from build123d import *

# Parameters (mm, degrees)
F8_DEPTH  = 16.5
F2_W      = 43
F2_H      = 66
F9_DEPTH  = 15
F4_W      = 6
F4_H      = 6
F4_H_2    = 5
F10_DEPTH = 16.5
F5_W      = 8
F5_H      = 6
F5_W_2    = 6
F5_H_2    = 8
F11_DEPTH = 4
F6_W      = 6
F6_H      = 10
F12_DEPTH = 3
F7_R      = 1.63195
F13_DEPTH = 16.501


with BuildPart() as f8:
    # F1 (on Front) → F8 (new body)
    with BuildSketch(Plane.XZ):
        Polygon((22.625, -32.5), (22.625, -24.5), (22.625, 36.5), (-23.375, 36.5), (-23.375, -32.5), align=None)
    extrude(amount=F8_DEPTH)

    # F2 (on Front) → F9 (cut)
    with BuildSketch(Plane.XZ):
        with Locations((-0.375, 2)):
            Rectangle(F2_W, F2_H)
    extrude(amount=F9_DEPTH, mode=Mode.SUBTRACT)

    # F4 (on Front) → F10 (join, through all)
    with BuildSketch(Plane.XZ):
        with Locations((-20.375, 33.5)):
            Rectangle(F4_W, F4_H)
        with Locations((19.625, 33.5)):
            Rectangle(F4_W, F4_H)
        with Locations((-0.375, -30)):
            Rectangle(F4_W, F4_H_2)
    extrude(amount=F10_DEPTH)

    # F5 (on Front) → F11 (cut)
    with BuildSketch(Plane.XZ):
        with Locations((-0.375, 33.5)):
            Rectangle(F5_W, F5_H)
        with Locations((-22.875, -3)):
            Rectangle(F5_W_2, F5_H_2)
    extrude(amount=F11_DEPTH, mode=Mode.SUBTRACT)

    # F6 (on Front) → F12 (cut)
    with BuildSketch(Plane.XZ):
        with Locations((-22.875, 12.5)):
            Rectangle(F6_W, F6_H)
        with Locations((-22.875, -18.5)):
            Rectangle(F6_W, F6_H)
        with Locations((22.125, 12.5)):
            Rectangle(F6_W, F6_H)
        with Locations((22.125, -18.5)):
            Rectangle(F6_W, F6_H)
    extrude(amount=F12_DEPTH, mode=Mode.SUBTRACT)

    # F7 (on Front) → F13 (cut, through all)
    with BuildSketch(Plane.XZ):
        with Locations((-0.375, -30)):
            Circle(F7_R)
        with Locations((-20.375, 33.5)):
            Circle(F7_R)
        with Locations((19.625, 33.5)):
            Circle(F7_R)
    extrude(amount=F13_DEPTH, mode=Mode.SUBTRACT)


solid = f8.part
Could you check a few things on this model? Use its own coordinates, in mm. A direction names the side the tool comes from. Give positions to 0.01 mm unless a question says otherwise; leave off trailing zeros. Order: outer loops, then holes, each group sorted by start corner. A loop starts at its lowest first (then second) coordinate and runs counter-clockwise, first axis right, second up. Notation, with made-up numbers: (45.5, -5.5) - (102.5, -5.5) arc R33 cw to (102.5, 23.5) - close; hole circle Ø8 at (88.25, 28). An arc over 180 degrees is marked (long way). One line per item, written item: value. Start each with the question number.
1. For faces 1 (the face through (-18, 0, 31)), 2 (the face through (22, -3, -18)), 3 (the face through (3.625, -2, 36)), 4 (the face through (21.125, -7, -1)), which set-ups out of +Z, -Z, +X, -X, +Y, -Y let a thin tool reach every point of the face, with its end or its side?
2. Imagine slicing it at A-A on z = 33.5. List the corners of the cut face in (x, y) for me (3 decimals), plus the area to 3 significant figures.
3. Imagine slicing it at D-D on z = -30. List the corners of the cut face in (x, y) for me (3 decimals), plus the area to 3 significant figures.
4. Imagine slicing it at B-B on x = 12. List the corners of the cut face in (y, z) for me, plus the area to 4 significant figures.
5. If I drill on probe 1 along X at (y, z) = (-3.5, -30) (3 decimals); probe 2 along X at (y, z) = (-7, 33.5) (3 decimals); probe 3 along Z at (x, y) = (11, -14.75), over which ranges is the centre line in solid material (lowest first)?
6. For P1, Ø8, axis at x = -15, z = -5, coming from the +Y side; P2, Ø1.2, axis at x = -23, z = -16, coming from the +Y side; P3, Ø1.2, axis at x = -23, z = -4, coming from the +Y side; P4, Ø3, axis at x = 19.625, z = 33.5, coming from the -Y side, each with a flat end and sliding along its axis, tell me the tip position at first contact or that it passes through.
7. Thinking about a two-plate mould opening in Z: for faces 5 (the face through (-23, 0, -10)), 6 (the face through (20.502, -8.134, 34.876)), which applies, +Z half, -Z half, draft (parallel to the pull), parting line (faces both ways), or undercut?
8. Imagine slicing it at C-C on y = -10.75. List the corners of the cut face in (x, z) for me (3 decimals).
Values:
1. face 1: +Z, -Z, +X, -X, +Y
1. face 2: +X, -X, +Y
1. face 3: +Z, +Y
1. face 4: +Y
2. outline: (-23.375, -16.5) - (-22.007, -16.5) - (-22.007, 0) - (-23.375, 0) - close; (-18.743, -16.5) - (17.993, -16.5) - (17.993, 0) - (16.625, 0) - (16.625, -15) - (-17.375, -15) - (-17.375, 0) - (-18.743, 0) - close; (21.257, -16.5) - (22.625, -16.5) - (22.625, 0) - (21.257, 0) - close
2. area: 141 mm²
3. outline: (-23.375, -16.5) - (-2.007, -16.5) - (-2.007, 0) - (-3.375, 0) - (-3.375, -15) - (-21.875, -15) - (-21.875, 0) - (-23.375, 0) - close; (1.257, -16.5) - (22.625, -16.5) - (22.625, 0) - (21.125, 0) - (21.125, -15) - (2.625, -15) - (2.625, 0) - (1.257, 0) - close
3. area: 150 mm²
4. outline: (-16.5, -32.5) - (0, -32.5) - (0, -31) - (-15, -31) - (-15, 35) - (0, 35) - (0, 36.5) - (-16.5, 36.5) - close
4. area: 148.5 mm²
5. probe 1: -23.375 to -21.875, -3.375 to -2.007, 1.257 to 2.625, 21.125 to 22.625
5. probe 2: -23.375 to -22.007, -18.743 to -17.375, 16.625 to 17.993, 21.257 to 22.625
5. probe 3: -32.5 to -31, 35 to 36.5
6. P1: y = -15
6. P2: y = -3
6. P3: y = -4
6. P4: through
7. face 5: draft
7. face 6: undercut
8. outline: (-23.375, -32.5) - (22.625, -32.5) - (22.625, 36.5) - (-23.375, 36.5) - close; hole circle Ø3.264 at (-20.375, 33.5); hole (-21.875, -31) - (-3.375, -31) - (-3.375, -27.5) - (2.625, -27.5) - (2.625, -31) - (21.125, -31) - (21.125, 30.5) - (16.625, 30.5) - (16.625, 35) - (-17.375, 35) - (-17.375, 30.5) - (-21.875, 30.5) - close; hole circle Ø3.264 at (-0.375, -30); hole circle Ø3.264 at (19.625, 33.5)
